from build123d import *

# Parameters (mm, degrees)
BOSS_EXTRUDE1_DEPTH = 40
SKETCH2_W           = 180
SKETCH2_H           = 50
CUT_EXTRUDE1_DEPTH  = 171.293863659
SKETCH3_R           = 17.5
BOSS_EXTRUDE3_DEPTH = 3
SKETCH4_R           = 30
BOSS_EXTRUDE4_DEPTH = 10
SKETCH5_R           = 25
BOSS_EXTRUDE5_DEPTH = 3
FILLET2_R           = 100
FILLET3_R           = 10
FILLET4_R           = 5


with BuildPart() as part:
    # Sketch1 → Boss-Extrude1 (new, symmetric)
    with BuildSketch(Plane.XY):
        with BuildLine():
            Line((0, 0), (94.268250808, 0))
            Line((94.268250808, 0), (125.20944533, 5.45576741))
            ThreePointArc((125.20944533, 5.45576741), (150, 35), (125.20944533, 64.54423259))
            Line((125.20944533, 64.54423259), (94.268250808, 70))
            Line((94.268250808, 70), (0, 70))
            Line((0, 70), (0, 0))
        make_face()
    extrude(amount=BOSS_EXTRUDE1_DEPTH, both=True)

    # Sketch2 → Cut-Extrude1 (cut, through all)
    with BuildSketch(Plane(origin=(0, 0, 0), x_dir=(1, 0, 0), z_dir=(0, 1, 0))):
        with Locations((110, 0)):
            Rectangle(SKETCH2_W, SKETCH2_H)
    extrude(amount=CUT_EXTRUDE1_DEPTH, mode=Mode.SUBTRACT)

    # Sketch3 → Boss-Extrude3 (add)
    with BuildSketch(Plane.XY.offset(-25)):
        with Locations((120, 35)):
            Circle(SKETCH3_R)
    boss_extrude3 = extrude(amount=BOSS_EXTRUDE3_DEPTH)

    # Mirror1: Boss-Extrude3 across plane
    add(boss_extrude3.mirror(Plane.XY))

    # Sketch4 → Boss-Extrude4 (add)
    with BuildSketch(Plane.ZY):
        with Locations((0, 35)):
            Circle(SKETCH4_R)
    extrude(amount=BOSS_EXTRUDE4_DEPTH)

    # Sketch5 → Boss-Extrude5 (add)
    with BuildSketch(Plane.ZY.offset(10)):
        with Locations((0, 35)):
            Circle(SKETCH5_R)
    extrude(amount=BOSS_EXTRUDE5_DEPTH)

    # Fillet2
    fillet2_edges = [part.edges().sort_by_distance(p)[0] for p in [
        (94.268250808, 70, 32.5),
        (94.268250808, 0, 32.5),
        (94.268250808, 70, -32.5),
        (94.268250808, 0, -32.5),
    ]]
    fillet(fillet2_edges, radius=FILLET2_R)

    # Fillet3
    fillet3_edges = [part.edges().sort_by_distance(p)[0] for p in [
        (20, 35, 25),
        (20, 35, -25),
    ]]
    fillet(fillet3_edges, radius=FILLET3_R)

    # Fillet4
    fillet4_edges = [part.edges().sort_by_distance(p)[0] for p in [
        (0, 0, 0),
        (150, 35, 40),
        (114.046823776, 66.512503946, 40),
        (150, 35, 25),
        (114.046823776, 3.487496054, 25),
        (150, 35, -25),
        (114.046823776, 66.512503946, -25),
        (0, 35, 40),
        (57.759692228, 70, -25),
        (42.759692228, 70, -40),
        (42.759692228, 70, 40),
        (114.046823776, 3.487496054, -40),
        (94.23495873, 0.380530191, -40),
        (94.23495873, 69.619469809, -40),
        (114.046823776, 3.487496054, -25),
        (57.759692228, 0, -25),
        (94.23495873, 0.380530191, -25),
        (94.23495873, 69.619469809, -25),
        (114.046823776, 66.512503946, 25),
        (94.23495873, 0.380530191, 25),
        (94.23495873, 69.619469809, 25),
        (114.046823776, 3.487496054, 40),
        (94.23495873, 0.380530191, 40),
        (94.23495873, 69.619469809, 40),
        (114.046823776, 66.512503946, -40),
        (150, 35, -40),
        (42.759692228, 0, -40),
        (20, 0, 0),
        (20, 70, 0),
        (0, 35, -40),
        (57.759692228, 70, 25),
        (57.759692228, 0, 25),
        (42.759692228, 0, 40),
        (22.928932188, 0, 22.071067812),
        (22.928932188, 70, 22.071067812),
        (22.928932188, 0, -22.071067812),
        (22.928932188, 70, -22.071067812),
    ]]
    fillet(fillet4_edges, radius=FILLET4_R - 0.0001)  # a hair under: the kernel refuses the full size


solid = part.part
Could you check a few things on this model? Use its own coordinates, in mm. A direction names the side the tool comes from. Give positions to 0.01 mm unless a question says otherwise; leave off trailing zeros. Loops run counter-clockwise (first coordinate to the right, second up) from the corner with the lowest first, then second, coordinate; pieces in that order, holes last. Notation, with made-up numbers: (18.25, 31) -> (57.25, 31) arc R18 ccw to (57.25, 65) -> close; hole circle Ø1 at (65.25, 55). An arc over 180 degrees is marked (long way). Answer as CSV lines item,"result". Start each with the question number.
(1) If we section it at D-D on z = -8.5: Write out the boundary of the cut face in (x, y).
(2) We'd pull the mould along Z, two halves only. Please class faces 1 (the cylindrical face through (136.69, 40.26, 23.52)), 2 (the cylindrical face through (1, 37, -38)), 3 (the cylindrical face through (2, 1, 0)), 4 (the cylindrical face through (113.942, 4.996, 38.574)): released by +Z, released by -Z, zero draft, split by the parting line, or undercut.
(3) I'm going to push flat-ended pins straight in: pin 1 Ø4 at (x, z) = (50.5, 28.5) entering from -Y; pin 2 Ø24 at (y, z) = (29, 2.5) entering from +X. Where does each tip first touch, or does it pass through?
(4) I need wall thicknesses on probe 1 along Z at (x, y) = (128.5, 52); probe 2 along Z at (x, y) = (25, 27.5); probe 3 along X at (y, z) = (18, 9.5). Which ranges of each line are inside material? Lowest first, please.
(5) Which directions (+Z, -Z, +X, -X, +Y, -Y) give clear straight access to the entire face, cutting with the end or side of a thin tool? Please do faces 5 (the cylindrical face through (22.85, 35.42, -21.99)), 6 (the flat face through (120, 35, -22)), 7 (the cylindrical face through (19, 68, 0)).
(6) If we section it at A-A on x = 32.5: Write out the boundary of the cut face in (y, z).
Computed:
1,outline,"(-13, 11.49) -> (-10, 11.49) -> (-10, 6.23) -> (0, 6.23) -> (0, 5) arc R5 ccw to (5, 0) -> (15, 0) arc R5 ccw to (20, 5) -> (20, 65) arc R5 ccw to (15, 70) -> (0, 70) -> (0, 63.77) -> (-10, 63.77) -> (-10, 58.51) -> (-13, 58.51) -> close"
2,face 1,"undercut"
2,face 2,"released by -Z"
2,face 3,"zero draft"
2,face 4,"released by +Z"
3,pin 1,"stops at y = 0"
3,pin 2,"stops at x = 20"
4,probe 1,"z = -40 to -25, 25 to 40"
4,probe 2,"z = -40 to -23.66, 23.66 to 40"
4,probe 3,"x = -13 to 20"
5,face 5,"+Y, -Y"
5,face 6,"+X, +Y, -Y"
5,face 7,"+X, +Y"
6,outline,"(0, -35) arc R5 ccw to (5, -40) -> (65, -40) arc R5 ccw to (70, -35) -> (70, -30) arc R5 ccw to (65, -25) -> (5, -25) arc R5 ccw to (0, -30) -> close; (0, 30) arc R5 ccw to (5, 25) -> (65, 25) arc R5 ccw to (70, 30) -> (70, 35) arc R5 ccw to (65, 40) -> (5, 40) arc R5 ccw to (0, 35) -> close"
